Drawing for the job (mm, zero at the part's lowest x, y, z). Coordinates: 2 decimals unless noted, no trailing zeros. Write each loop counter-clockwise with the first axis right and the second up, starting at its lowest first coordinate (ties: lowest second). Pieces come first, ordered by that corner, then holes. Notation, with made-up numbers: (-5, 26.25) -> (37, 26.25) arc R26 ccw to (37, 43.25) -> close; hole circle Ø8 at (-24.5, -33). An arc over 180 degrees is marked (long way). Answer as CSV lines item,"result".
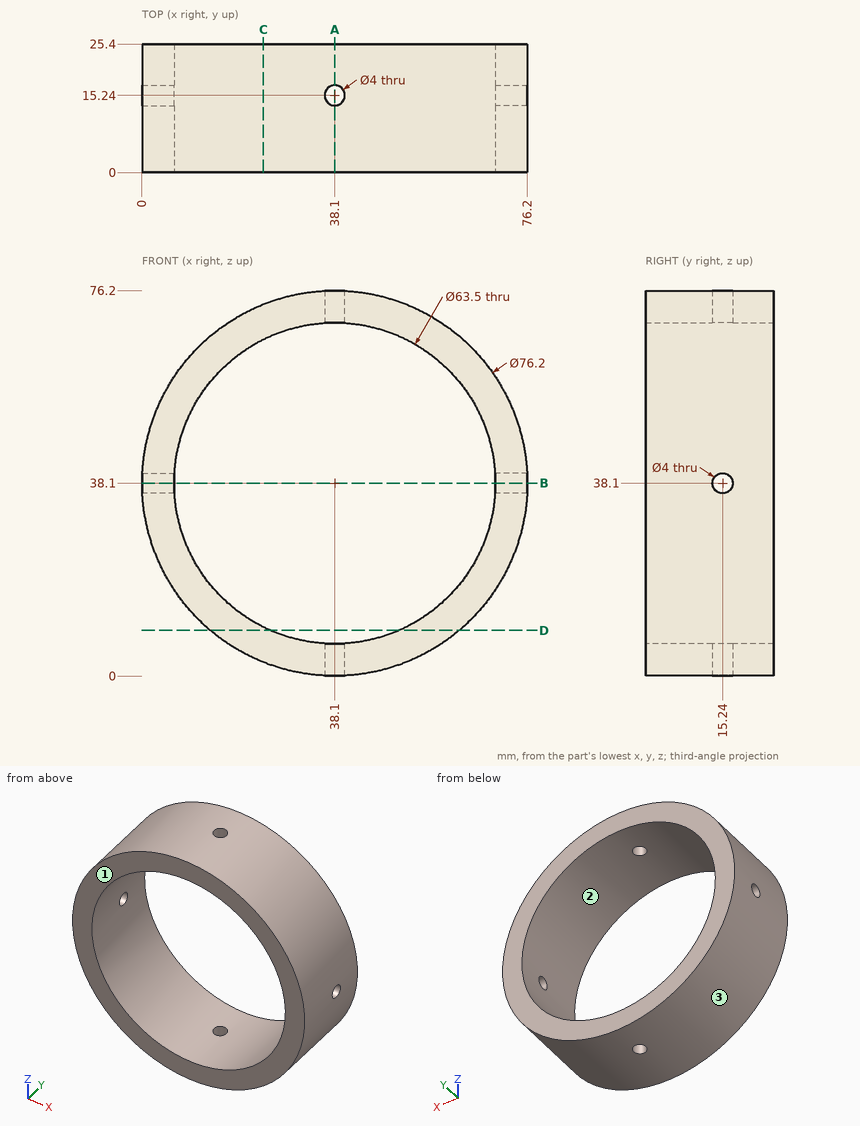
Item 1: Saw through at A-A on x = 38.1. Give the cut face in (y, z), and give its area (3 significant figures).
Answer below:
outline,"(0, 0) -> (13.24, 0) -> (13.24, 6.35) -> (0, 6.35) -> close; (0, 69.85) -> (13.24, 69.85) -> (13.24, 76.2) -> (0, 76.2) -> close; (17.24, 0) -> (25.4, 0) -> (25.4, 6.35) -> (17.24, 6.35) -> close; (17.24, 69.85) -> (25.4, 69.85) -> (25.4, 76.2) -> (17.24, 76.2) -> close"
area,"272 mm2"
Item 2: Wall check: line 1 (Y direction, x = 38, z = 74); line 2 (X direction, y = 12.25, z = 38.1); line 3 (Z direction, x = 59.5, y = 3.5). Give the ranges that are in metal, low to high. Write a range as from..to.
Answer below:
line 1,"y = 0..13.24, 17.24..25.4"
line 2,"x = 0..6.35, 69.85..76.2"
line 3,"z = 6.58..14.65, 61.55..69.62"
Item 3: Two-plate mould, pull along X, no slides. Class the marked faces 1, 2 and 3: pulls with the +X half, pulls with the -X half, needs draft (parallel to the pull), parting line crosses it, or undercut.
Answer below:
face 1,"needs draft"
face 2,"undercut"
face 3,"parting line crosses it"
Item 4: Saw through at B-B on z = 38.1. Give the cut face in (x, y), and give its area (3 significant figures).
Answer below:
outline,"(0, 0) -> (6.35, 0) -> (6.35, 13.24) -> (0, 13.24) -> close; (0, 17.24) -> (6.35, 17.24) -> (6.35, 25.4) -> (0, 25.4) -> close; (69.85, 0) -> (76.2, 0) -> (76.2, 13.24) -> (69.85, 13.24) -> close; (69.85, 17.24) -> (76.2, 17.24) -> (76.2, 25.4) -> (69.85, 25.4) -> close"
area,"272 mm2"
Item 5: Saw through at D-D on z = 9. Give the cut face in (x, y).
Answer below:
outline,"(13.51, 0) -> (25.4, 0) -> (25.4, 25.4) -> (13.51, 25.4) -> close; (50.8, 0) -> (62.69, 0) -> (62.69, 25.4) -> (50.8, 25.4) -> close"
Item 6: Saw through at C-C on x = 24. Give the cut face in (y, z), and give its area (3 significant figures).
Answer below:
outline,"(0, 2.71) -> (25.4, 2.71) -> (25.4, 9.65) -> (0, 9.65) -> close; (0, 66.55) -> (25.4, 66.55) -> (25.4, 73.49) -> (0, 73.49) -> close"
area,"353 mm2"
Item 7: Flat gauge pins, fed straight in: pin 1 (3 mm diameter, centred on x = 53, y = 10, fed in from -Z); pin 2 (4 mm diameter, centred on x = 54.5, y = 18, fed in from +Z); pin 3 (3.5 mm diameter, centred on x = 38.1, y = 15.24, fed in from +Z); pin 4 (4 mm diameter, centred on x = 53.5, y = 11.5, fed in from +Z). Where does each tip first touch, or does it go through?
Answer below:
pin 1,"stops at z = 2.43"
pin 2,"stops at z = 73.37"
pin 3,"passes through"
pin 4,"stops at z = 73.77"
